from build123d import *

# Parameters (mm, degrees)
SKETCH1_R             = 44.5
BOSS_EXTRUDE2_DEPTH   = 3
SKETCH3_R             = 44.5
SKETCH3_R_2           = 41.5
BOSS_EXTRUDE3_DEPTH   = 10
SKETCH4_R             = 57.5
SKETCH4_R_2           = 41.5
BOSS_EXTRUDE4_DEPTH   = 3
SKETCH5_R             = 22.5
CUT_EXTRUDE1_DEPTH    = 83.349863388
FILLET1_R             = 3
FILLET2_R             = 5
F_1_0MM_DOWEL_HOLE2_D = 6.6
CIRPATTERN2_COUNT     = 6


with BuildPart() as part:
    # Sketch1 → Boss-Extrude2 (new body)
    with BuildSketch(Plane(origin=(0, 0, 0), x_dir=(0, 0, -1), z_dir=(1, 0, 0))):
        Circle(SKETCH1_R)
    extrude(amount=BOSS_EXTRUDE2_DEPTH)

    # Sketch3 → Boss-Extrude3 (add)
    with BuildSketch(Plane(origin=(3, 0, 0), x_dir=(0, 0, -1), z_dir=(1, 0, 0))):
        Circle(SKETCH3_R)
        Circle(SKETCH3_R_2, mode=Mode.SUBTRACT)
    extrude(amount=BOSS_EXTRUDE3_DEPTH)

    # Sketch4 → Boss-Extrude4 (add)
    with BuildSketch(Plane(origin=(13, 0, 0), x_dir=(0, 0, -1), z_dir=(1, 0, 0))):
        Circle(SKETCH4_R)
        Circle(SKETCH4_R_2, mode=Mode.SUBTRACT)
    extrude(amount=BOSS_EXTRUDE4_DEPTH)

    # Sketch5 → Cut-Extrude1 (cut, through all)
    with BuildSketch(Plane(origin=(3, 0, 0), x_dir=(0, 0, -1), z_dir=(1, 0, 0))):
        Circle(SKETCH5_R)
    extrude(amount=-CUT_EXTRUDE1_DEPTH, mode=Mode.SUBTRACT)

    # Fillet1
    fillet1_edges = [part.edges().sort_by_distance(p)[0] for p in [
        (3, 0, 41.5),
    ]]
    fillet(fillet1_edges, radius=FILLET1_R)

    # Fillet2
    fillet2_edges = [part.edges().sort_by_distance(p)[0] for p in [
        (0, 0, 44.5),
    ]]
    fillet(fillet2_edges, radius=FILLET2_R)

    # Ø1.0mm Dowel Hole2 (through all)
    with Locations(Plane(origin=(3, 0, 0), x_dir=(0, 0, -1), z_dir=(1, 0, 0))):
        with Locations((0, 32)):
            f_1_0mm_dowel_hole2 = Hole(F_1_0MM_DOWEL_HOLE2_D / 2)

    # CirPattern2: Ø1.0mm Dowel Hole2 ×6 about axis
    cirpattern2_axis = Axis((0, 0, 0), (1, 0, 0))
    for i in range(1, CIRPATTERN2_COUNT):
        add(f_1_0mm_dowel_hole2.rotate(cirpattern2_axis, i * 360 / CIRPATTERN2_COUNT), mode=Mode.SUBTRACT)


solid = part.part
Work out the finished part from the listing and answer in its coordinate system (mm). A direction names the side the tool comes from. Coordinates: 2 decimals unless noted, no trailing zeros. Write each loop counter-clockwise with the first axis right and the second up, starting at its lowest first coordinate (ties: lowest second). Pieces come first, ordered by that corner, then holes.
1. Flat-ended cylindrical pins translate along their axes: pin 1 (10.5 mm diameter, centred on y = -16, z = -27.71, fed in from -X); pin 2 (2 mm diameter, centred on x = 4.5, z = 21.5, fed in from +Y); pin 3 (5 mm diameter, centred on y = 42, z = -44.5, fed in from +X); pin 4 (6 mm diameter, centred on x = 8, z = -13.5, fed in from -Y). Find the tip coordinate at first contact, or state that the pin passes through.
Results list:
pin 1: stops at x = 0
pin 2: stops at y = 39.48
pin 3: passes through
pin 4: stops at y = -43.24
2. For a pull along Y with two mould halves and no side action, classify faces 1 (the flat face through (16, 17.3, -38.1)), 2 (the cylindrical face through (1.479, -17.264, 30.761)), 3 (the cylindrical face through (8.944, 30.075, 32.798)) as +Y half, -Y half, draft (parallel to the pull), parting line (faces both ways), or undercut.
Results list:
face 1: draft
face 2: undercut
face 3: parting line
3. The part is cut by section A-A, the plane z = 0. Write down the section's boundary in (x, y), and give its area (3 significant figures).
Results list:
outline: (0, -39.5) arc R5 ccw to (5, -44.5) - (13, -44.5) - (13, -57.5) - (16, -57.5) - (16, -41.5) - (6, -41.5) arc R3 cw to (3, -38.5) - (3, -35.3) - (0, -35.3) - close; (0, -28.7) - (3, -28.7) - (3, -22.5) - (0, -22.5) - close; (0, 22.5) - (3, 22.5) - (3, 28.7) - (0, 28.7) - close; (0, 35.3) - (3, 35.3) - (3, 38.5) arc R3 cw to (6, 41.5) - (16, 41.5) - (16, 57.5) - (13, 57.5) - (13, 44.5) - (5, 44.5) arc R5 ccw to (0, 39.5) - close
area: 242 mm2
4. Consider line 1 along Y through (x, z) = (1.9, 0); line 2 along X through (y, z) = (6, 48.5); line 3 along X through (y, z) = (9, -31.5). Determine where each line is inside the solid, lowest interval first.
Results list:
line 1: y = -43.42 to -35.3, -28.7 to -22.5, 22.5 to 28.7, 35.3 to 43.42
line 2: x = 13 to 16
line 3: x = 0 to 3
5. The part is cut by section B-B, the plane y = 0. Write down the section's boundary in (x, z).
Results list:
outline: (0, -39.5) arc R5 ccw to (5, -44.5) - (13, -44.5) - (13, -57.5) - (16, -57.5) - (16, -41.5) - (6, -41.5) arc R3 cw to (3, -38.5) - (3, -22.5) - (0, -22.5) - close; (0, 22.5) - (3, 22.5) - (3, 38.5) arc R3 cw to (6, 41.5) - (16, 41.5) - (16, 57.5) - (13, 57.5) - (13, 44.5) - (5, 44.5) arc R5 ccw to (0, 39.5) - close
6. For faces 4 (the flat face through (13, -34, -30)), 5 (the cylindrical face through (1.521, -19.961, -10.382)), 6 (the cylindrical face through (10.93, 12.465, -39.584)), determine the directions among +Z, -Z, +X, -X, +Y, -Y from which every point of the face is accessible in a straight line to the end or side of a thin tool.
Results list:
face 4: -X
face 5: +X, -X
face 6: +X
7. The part is cut by section D-D, the plane y = 50. Write down the section's boundary in (x, z), and give its area (3 significant figures).
Results list:
outline: (13, -28.39) - (16, -28.39) - (16, 28.39) - (13, 28.39) - close
area: 170 mm2
8. The part is cut by section C-C, the plane x = 10.75. Write down the section's boundary in (y, z), and give its area (3 significant figures).
Results list:
outline: circle Ø89 at (0, 0); hole circle Ø83 at (0, 0)
area: 811 mm2
